Solid Edge part; units mm, degrees
sketch "Sketch1" plane through (0, 0, 0) normal (0, 0, 1) x (1, 0, 0)
  line L0 (-50.4769, -0.1262) -> (-31.3427, -46.3202)
  line L1 (-31.3427, -46.3202) -> (-10.2002, -25.1777)
  line L2 (-10.2002, -25.1777) -> (-24.3402, -25.1777)
  line L3 (-24.3402, -25.1777) -> (26.5942, 25.7567)
  line L4 (26.5942, 25.7567) -> (19.5231, 32.8278)
  line L5 (19.5231, 32.8278) -> (-26.4388, -13.1341)
  line L6 (-26.4388, -13.1341) -> (-50.4769, -0.1262)
  dimension "D1" = 50.4769
  dimension "D2" = 31.3427
  dimension "D3" = 26.5942
  dimension "D4" = 19.5231
  dimension "D5" = 10.2002
extrude "Protrusion1" add sketch "Sketch1" along normal blind 35
sketch "Sketch2" plane through (-12.0121, -6.8169, 0) normal (0, 0, -1) x (-0.8795, 0.4759, 0)
  line L0 (-1.7996, -43.9425) -> (-10.3318, -15.2857)
  line L1 (-10.3318, -15.2857) -> (2.1041, -22.0153)
  line L2 (2.1041, -22.0153) -> (-18.451, 47.0217)
  line L3 (-18.451, 47.0217) -> (6.4693, 54.4415)
  line L4 (6.4693, 54.4415) -> (28.4484, -19.3779)
  line L5 (28.4484, -19.3779) -> (-1.7996, -43.9425)
extrude "Extrusionsausprägung_6" add sketch "Sketch2" against normal blind 4
sketch "Sketch3" plane through (-3.4579, 9.8468, 19.5) normal (-0.7071, 0.7071, 0) x (0, 0, 1)
  circle A0 centre (-6.5, 10.45) radius 3.5
  circle A1 centre (-6.5, -19.55) radius 3.5
  dimension "D1" = 6.5
extrude "Cutout1" cut sketch "Sketch3" against normal through all
chamfer "Fase_3" distance 3 angle 45 2 edges at (-20.7715, -35.7489, 0) (1.127, 0.2895, 0)
properties material "Nylon, allgemein"
For this review, take the finished solid that the model builds, in its own axes (mm). A direction names the side the tool comes from. Round coordinates to 2 decimals unless told otherwise and drop trailing zeros. Loops run counter-clockwise (first coordinate to the right, second up) from the corner with the lowest first, then second, coordinate; pieces in that order, holes last. Notation, with made-up numbers: (76.25, 28.5) - (107.25, 28.5) arc R18 ccw to (107.25, 53.5) - close; hole circle Ø2 at (89, 54). An arc over 180 degrees is marked (long way). One line per item, written item: value. Start each with the question number.
Item 1: For L1, parallel to Y at x = -24, z = 32; L2, parallel to Y at x = -17.5, z = 26; L3, parallel to X at y = -13, z = 15.5, list the stretches that pass through material, from the lowest coordinate up.
Item 2: The part is to be moulded in two halves that separate along Y. For faces 1 (the flat face through (-21.965, -34.852, 1.521)), 2 (the flat face through (-38.29, -6.72, 17.26)), 3 (the cylindrical face through (-15.991, -9.659, 14.615)), say which applies: +Y half, -Y half, draft (parallel to the pull), parting line (faces both ways), or undercut.
Item 3: Take a section at A-A (z = 18.5). Give the boundary of the cut face in (x, y).
Item 4: Take a section at C-C (z = 11.5). Give the boundary of the cut face in (x, y).
Item 5: Take a section at D-D (x = -38.5). Give the boundary of the cut face in (y, z), plus the area to 3 significant figures.
Item 6: Clearance check with flat-ended pins moving along their axes: pin 1 Ø10 at (y, z) = (15.5, 18) entering from +X; pin 2 Ø10 at (x, z) = (-24.5, 29.5) entering from +Y; pin 3 Ø2 at (x, z) = (-24, 19) entering from -Y. State where each tip first meets the part, or that it passes through.
Item 7: For faces 4 (the flat face through (23.11, 29.24, 17.26)), 5 (the flat face through (-11, 16, 4)), list the 3-axis set-ups (+Z, -Z, +X, -X, +Y, -Y) from which the entire face can be reached by the end or side of a thin tool; tool diameter is ignored.
Answer below:
1. L1: y = -38.98 to -25.18, -24.84 to -10.7
1. L2: y = -32.48 to -25.18, -18.34 to -4.2
1. L3: x = -45.14 to -26.69, -26.3 to -12.16
2. face 1: -Y half
2. face 2: +Y half
2. face 3: undercut
3. outline: (-50.48, -0.13) - (-31.34, -46.32) - (-10.2, -25.18) - (-24.34, -25.18) - (26.59, 25.76) - (19.52, 32.83) - (-26.44, -13.13) - close
4. outline: (-50.48, -0.13) - (-31.34, -46.32) - (-10.2, -25.18) - (-24.34, -25.18) - (-12.45, -13.28) - (-19.52, -6.21) - (-26.44, -13.13) - close; (-15.05, -1.74) - (-7.97, -8.81) - (8.77, 7.93) - (1.7, 15) - close; (6.17, 19.47) - (13.24, 12.4) - (26.59, 25.76) - (19.52, 32.83) - close
5. outline: (-29.04, 0) - (-2.57, 0) - (-2.57, 4) - (-6.61, 4) - (-6.61, 35) - (-29.04, 35) - close
5. area: 801 mm2
6. pin 1: stops at x = 21.34
6. pin 2: stops at y = -6.2
6. pin 3: stops at y = -39.98
7. face 4: +Z, -Z, +X, +Y
7. face 5: +Z, +Y
